```python
from build123d import *

# Parameters (mm, degrees)
F2_DEPTH  = 12.7
F1_R      = 1.5875
F3_DEPTH  = 4.7625
F4_R      = 1.5875
F5_DEPTH  = 15.859309
F9_W      = 1.5875
F9_H      = 9.525
F10_DEPTH = 25.4
F12_R     = 5.08


with BuildPart() as f2:
    # F0 (on Top) → F2 (new body)
    with BuildSketch(Plane.XY):
        with BuildLine():
            Line((-5.552635, 5.67205), (-5.552635, 8.681886))
            ThreePointArc((-5.552635, 8.681886), (0, -10.305673), (5.552635, 8.681886))
            Line((5.552635, 8.681886), (5.552635, 5.67205))
            ThreePointArc((5.552635, 5.67205), (7.317033, 3.076513), (7.9375, 0))
            ThreePointArc((7.9375, 0), (-3.076513, -7.317033), (-5.552635, 5.67205))
        make_face()
        with BuildLine():
            Line((-5.552635, 19.361428), (-5.552635, 8.681886))
            Line((-5.552635, 8.681886), (-5.552635, 5.67205))
            ThreePointArc((-5.552635, 5.67205), (-4.520661, 6.52438), (-3.360147, 7.191197))
            Line((-3.360147, 7.191197), (-3.360147, 19.361428))
            Line((-3.360147, 19.361428), (-5.552635, 19.361428))
        make_face()
        with BuildLine():
            Line((5.552635, 5.67205), (5.552635, 8.681886))
            Line((5.552635, 8.681886), (5.552635, 19.361428))
            Line((5.552635, 19.361428), (3.360147, 19.361428))
            Line((3.360147, 19.361428), (3.360147, 7.191197))
            ThreePointArc((3.360147, 7.191197), (4.520661, 6.52438), (5.552635, 5.67205))
        make_face()
    extrude(amount=F2_DEPTH)

    # F1 (on Right) → F3 (join, symmetric)
    with BuildSketch(Plane.YZ):
        with BuildLine():
            Line((-7.938393, 9.522529), (-14.914774, 9.522529))
            ThreePointArc((-14.914774, 9.522529), (-19.830673, 4.7625), (-14.914774, 0.002471))
            Line((-14.914774, 0.002471), (-14.914774, 0))
            Line((-14.914774, 0), (-7.938393, 0))
            Line((-7.938393, 0), (-7.938393, 9.522529))
        make_face()
        with Locations((-15.068173, 4.7625)):
            Circle(F1_R, mode=Mode.SUBTRACT)
    extrude(amount=F3_DEPTH, both=True)

    # F4 (on face) → F5 (cut, through all)
    with BuildSketch(Plane.YZ.offset(5.552635)):
        with Locations((14.021657, 6.35)):
            Circle(F4_R)
    extrude(amount=-F5_DEPTH, mode=Mode.SUBTRACT)


with BuildPart() as f6_1:
    # F6: copy of F2
    add(f2.part)


with BuildPart() as f8_1:
    # F8: copy of F2
    add(f2.part)


with BuildPart() as f10_tool:
    # F9 (on Top) → F10 (new body)
    with BuildSketch(Plane.XY):
        with Locations((0.79375, -15.068173)):
            Rectangle(F9_W, F9_H)
        with Locations((-0.79375, -15.068173)):
            Rectangle(F9_W, F9_H)
    extrude(amount=F10_DEPTH)


with BuildPart() as f2_1:
    add(f2.part)

    # F10: cut by f10_tool
    add(f10_tool.part, mode=Mode.SUBTRACT)


with BuildPart() as f8_1_1:
    add(f8_1.part)

    # F10: cut by f10_tool
    add(f10_tool.part, mode=Mode.SUBTRACT)

    # F12
    f12_edges = [f8_1_1.edges().sort_by_distance(p)[0] for p in [
        (-4.456391, 19.361428, 12.7),
        (4.456391, 19.361428, 12.7),
        (-4.456391, 19.361428, 0),
        (4.456391, 19.361428, 0),
    ]]
    fillet(f12_edges, radius=F12_R)


solid = f8_1_1.part
```
Check sheet for the modelled part. Datum: model origin and axes. Units: mm. A direction names the side the tool comes from. Round coordinates to 2 decimals unless told otherwise and drop trailing zeros. Order: outer loops, then holes, each group sorted by start corner. A loop starts at its lowest first (then second) coordinate and runs counter-clockwise, first axis right, second up. Notation, with made-up numbers: (65, 57) - (103, 57) arc R25 ccw to (103, 75) - close; hole circle Ø5 at (50, 42). An arc over 180 degrees is marked (long way). Write item = value, one per line.
Q1. Draft check along Y on faces 5 (the face through (-4.472, 17.834, 1.449)), 6 (the face through (5, 7, 12.7)), 7 (the face through (3.153, -16.654, 4.832)). Enter one of: pulls with the +Y half, pulls with the -Y half, needs draft (parallel to the pull), parting line crosses it, or undercut.
Computed:
face_5 = pulls with the +Y half
face_6 = needs draft
face_7 = undercut
Q2. Tool access check on faces 1 (the face through (-1.588, -13, 5)), 2 (the face through (5.553, 13, 8)), 3 (the face through (3.36, 12, 6)), 4 (the face through (-4.54, 6.51, 6.26)). Record the directions out of +Z, -Z, +X, -X, +Y, -Y that give a thin tool (end or side, any length) a straight path to the whole face; none if there is none.
Computed:
face_1 = +Z, -Z, -Y
face_2 = +Z, -Z, +X, +Y
face_3 = +Z, -Z, +Y
face_4 = +Z, -Z
Q3. Section check A-A (y = 11). Record the boundary of the cut face in (x, z), and give its area (3 significant figures).
Computed:
outline = (-5.55, 0) - (-3.36, 0) - (-3.36, 12.7) - (-5.55, 12.7) - close; (3.36, 0) - (5.55, 0) - (5.55, 12.7) - (3.36, 12.7) - close
area = 55.7 mm^2
Q4. Section check D-D (y = -11). Record the boundary of the cut face in (x, z), and give its area (3 significant figures).
Computed:
outline = (-4.76, 0) - (-1.59, 0) - (-1.59, 9.52) - (-4.76, 9.52) - close; (1.59, 0) - (4.76, 0) - (4.76, 9.52) - (1.59, 9.52) - close
area = 60.5 mm^2
Q5. Section check B-B (z = 4). Record the boundary of the cut face in (x, y) (1 decimal), and give its area (3 significant figures).
Computed:
outline = (-5.6, 5.7) arc R7.9 cw to (-3.4, 7.2) - (-3.4, 19.2) - (-5.6, 19.2) - (-5.6, 8.7) arc R10.3 ccw to (-4.8, -9.1) - (-4.8, -13.7) - (-1.6, -13.7) - (-1.6, -10.3) - (1.6, -10.3) - (1.6, -13.7) - (4.8, -13.7) - (4.8, -9.1) arc R10.3 ccw to (5.6, 8.7) - (5.6, 19.2) - (3.4, 19.2) - (3.4, 7.2) arc R7.9 cw to (5.6, 5.7) arc R7.9 cw to (7.9, 0) arc R7.9 cw (long way) to start; (-4.8, -19.8) - (-1.6, -19.8) - (-1.6, -16.5) - (-4.8, -16.5) - close; (1.6, -19.8) - (4.8, -19.8) - (4.8, -16.5) - (1.6, -16.5) - close
area = 209 mm^2
Q6. Thickness scan on line 1 along X through (y, z) = (16, 7.75); line 2 along X through (y, z) = (-11, 4.75); line 3 along Y through (x, z) = (-3.75, 5.5). Record the ranges inside material, lowest first.
Computed:
line_1 = -5.55 to -3.36, 3.36 to 5.55
line_2 = -4.76 to -1.59, 1.59 to 4.76
line_3 = -19.77 to -16.47, -13.66 to -7, 7 to 12.68, 15.36 to 19.36
Q7. Section check C-C (y = 15). Record the boundary of the cut face in (x, z), and give its area (3 significant figures).
Computed:
outline = (-5.55, 0.05) - (-3.36, 0.05) - (-3.36, 5.1) - (-5.55, 5.1) - close; (-5.55, 7.6) - (-3.36, 7.6) - (-3.36, 12.65) - (-5.55, 12.65) - close; (3.36, 0.05) - (5.55, 0.05) - (5.55, 5.1) - (3.36, 5.1) - close; (3.36, 7.6) - (5.55, 7.6) - (5.55, 12.65) - (3.36, 12.65) - close
area = 44.3 mm^2
Q8. Go/stop test with flat-tipped pins: pin 1 (7.5 mm diameter, centred on y = -13.5, z = 2.5, fed in from -X); pin 2 (12 mm diameter, centred on x = 4.5, y = -14.5, fed in from +Z); pin 3 (2.5 mm diameter, centred on x = 0.5, z = 5.5, fed in from -Y); pin 4 (1.5 mm diameter, centred on y = 11, z = 7, fed in from -X). Record where each tip stops, or that it passes through.
Computed:
pin_1 = -4.76
pin_2 = 12.7
pin_3 = -19.83
pin_4 = -5.55
